Design review of the part shown in the three views and the two pictorial views. Dimensions are in mm from the part's minimum x, y and z. A direction names the side the tool comes from. Round coordinates to 2 decimals unless told otherwise and drop trailing zeros. Loops run counter-clockwise (first coordinate to the right, second up) from the corner with the lowest first, then second, coordinate; pieces in that order, holes last. Notation, with made-up numbers: M -28.5,48 L 13.5,48 A9 cw 13.5,57 Z; hole C 74.25,26 d4. An arc over 180 degrees is marked long. Answer as CSV lines item,"result". Start each with the question number.
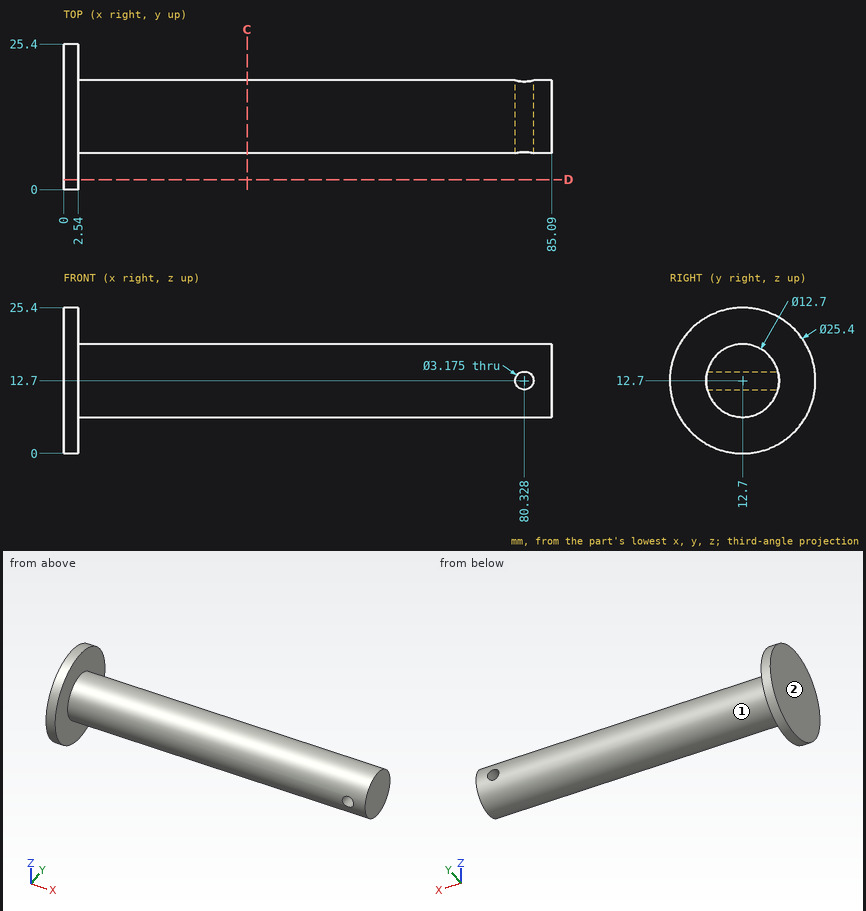
Item 1: Tool access review of the marked faces 1 and 2: name each direction out of +Z, -Z, +X, -X, +Y, -Y from which nothing blocks a thin tool from reaching the whole face with its end or side.
Item 2: Insertion check: pin 1 Ø4 at (x, y) = (18, 17) entering from +Z; pin 2 Ø6 at (x, y) = (46, 15.5) entering from -Z; pin 3 Ø3.5 at (x, z) = (80.33, 12.7) entering from +Y. Each pin has a flat end and moves straight along its axis. Give the tip position at first contact, or say it passes through.
Item 3: Consider section C-C, the plane x = 32. Write out the cut boundary in (y, z), then the cut area to 3 significant figures.
Item 4: To check wall thickness, follow line 1 (X direction, y = 15.25, z = 12.7) (1 decimal); line 2 (X direction, y = 17.25, z = 23.75); line 3 (Y direction, x = 25, z = 12.75). State the ranges of each line that lie inside material, in increasing order.
Item 5: Consider section D-D, the plane y = 1.75. Write out the cut boundary in (x, z), then the cut area to 3 significant figures.
Found:
1,face 1,"+X"
1,face 2,"+Z, -Z, -X, +Y, -Y"
2,pin 1,"stops at z = 18.62"
2,pin 2,"stops at z = 6.35"
2,pin 3,"stops at y = 19.05"
3,outline,"C 12.7,12.7 d12.7"
3,area,"127 mm^2"
4,line 1,"x = 0 to 78.7, 81.9 to 85.1"
4,line 2,"x = 0 to 2.54"
4,line 3,"y = 6.35 to 19.05"
5,outline,"M 0,6.27 L 2.54,6.27 L 2.54,19.13 L 0,19.13 Z"
5,area,"32.7 mm^2"
